Can you work these out from the model? Positions are in its coordinate system, mm. A direction names the side the tool comes from. Round coordinates to 2 decimals unless told otherwise and drop trailing zeros. Loops run counter-clockwise (first coordinate to the right, second up) from the corner with the lowest first, then second, coordinate; pieces in that order, holes last.
(1) Thinking about a two-plate mould opening in Z: for faces 1 (the face through (0.493, 13.631, 199.503)), 2 (the face through (5.6, 0.4, 251)), 3 (the face through (0.493, 13.631, 149.503)), 4 (the face through (10, 0, 124)), which applies, released by +Z, released by -Z, zero draft, split by the parting line, or undercut?
(2) If I drill on line 1 along X through (y, z) = (0.8, 134); line 2 along X through (y, z) = (0.2, 170); line 3 along X through (y, z) = (3.75, 181), over which ranges is the centre line in solid material (lowest first)?
(3) Will these pins go through, and if not, where does the flat tip stop? pin 1 Ø12 at (x, z) = (2.5, 29.5) entering from +Y; pin 2 Ø3 at (x, z) = (8.5, 128.5) entering from +Y; pin 3 Ø1 at (y, z) = (10, 103) entering from +X.
(4) I want a section at C-C on x = 17. Write out the boundary of the cut face in (y, z).
(5) I want a section at A-A on z = 10. Write out the boundary of the cut face in (x, y).
(6) Which directions (+Z, -Z, +X, -X, +Y, -Y) give clear straight access to the entire face, cutting with the end or side of a thin tool? Please do faces 5 (the face through (0.493, 15.082, 43.227)), 6 (the face through (1, 11, 124)).
(7) I want a section at B-B on z = 184. Write out the boundary of the cut face in (x, y), plus the area to 3 significant figures.
from build123d import *

# Parameters (mm, degrees)
EXTRUDE_1_DEPTH     = 251
SKETCH_3_R          = 1.5
SKETCH_3_R_2        = 1.6
CUT_EXTRUDE_1_DEPTH = 2
SKETCH_4_R          = 2.1
CUT_EXTRUDE_2_DEPTH = 21
SKETCH_5_R          = 2.25
CUT_EXTRUDE_3_DEPTH = 2


with BuildPart() as part:
    # Эскиз1 → Бобышка-Вытянуть1 (new body)
    with BuildSketch(Plane.XY):
        Polygon((0, 0), (0, 20), (1, 20), (1, 1), (20, 1), (20, 0), align=None)
    extrude(amount=EXTRUDE_1_DEPTH)

    # Эскиз3 → Вырез-Вытянуть1 (cut, through all)
    with BuildSketch(Plane(origin=(0, 1, 0), x_dir=(1, 0, 0), z_dir=(0, 1, 0))):
        with Locations((10.5, -134)):
            Circle(SKETCH_3_R)
        with Locations((10.5, -170)):
            Circle(SKETCH_3_R_2)
        with Locations((10.5, -66)):
            Circle(SKETCH_3_R_2)
        with Locations((10.5, -30)):
            Circle(SKETCH_3_R)
    extrude(amount=-CUT_EXTRUDE_1_DEPTH, mode=Mode.SUBTRACT)

    # Эскиз4 → Вырез-Вытянуть2 (cut, through all)
    with BuildSketch(Plane.ZY):
        with Locations((43.5, 13)):
            Circle(SKETCH_4_R)
        with Locations((93.5, 13)):
            Circle(SKETCH_4_R)
        with Locations((147.5, 13)):
            Circle(SKETCH_4_R)
        with Locations((197.5, 13)):
            Circle(SKETCH_4_R)
    extrude(amount=-CUT_EXTRUDE_2_DEPTH, mode=Mode.SUBTRACT)

    # Эскиз5 → Вырез-Вытянуть3 (cut, through all)
    with BuildSketch(Plane(origin=(0, 1, 0), x_dir=(1, 0, 0), z_dir=(0, 1, 0))):
        with Locations((10.5, -10)):
            Circle(SKETCH_5_R)
        with Locations((10.5, -241)):
            Circle(SKETCH_5_R)
    extrude(amount=-CUT_EXTRUDE_3_DEPTH, mode=Mode.SUBTRACT)


solid = part.part
Filled sheet:
1. face 1: undercut
1. face 2: released by +Z
1. face 3: undercut
1. face 4: zero draft
2. line 1: x = 0 to 9, 12 to 20
2. line 2: x = 0 to 8.9, 12.1 to 20
2. line 3: x = 0 to 1
3. pin 1: stops at y = 20
3. pin 2: stops at y = 1
3. pin 3: stops at x = 1
4. outline: (0, 0) - (1, 0) - (1, 251) - (0, 251) - close
5. outline: (0, 0) - (8.25, 0) - (8.25, 1) - (1, 1) - (1, 20) - (0, 20) - close; (12.75, 0) - (20, 0) - (20, 1) - (12.75, 1) - close
6. face 5: +X, -X
6. face 6: +Z, -Z, +X, +Y
7. outline: (0, 0) - (20, 0) - (20, 1) - (1, 1) - (1, 20) - (0, 20) - close
7. area: 39.0 mm2
